Source: CAD feature listing. Evaluate the final solid. Frame: model axes, mm. A direction names the side the tool comes from. Give positions to 0.01 mm unless a question says otherwise; leave off trailing zeros. Write each loop counter-clockwise with the first axis right and the second up, starting at its lowest first coordinate (ties: lowest second). Pieces come first, ordered by that corner, then holes. Notation, with made-up numbers: M 10.25,85.5 L 58.25,85.5 A25 cw 58.25,107.5 Z; hole C 83,4 d4. An arc over 180 degrees is marked long. Answer as a JSON object with one key per item and string values. Group by question number.
```python
from build123d import *

# Parameters (mm, degrees)
SKETCH1_R           = 40
SKETCH1_R_2         = 25
BOSS_EXTRUDE1_DEPTH = 30
BOSS_EXTRUDE2_DEPTH = 17
SKETCH3_R           = 17.5
CUT_EXTRUDE1_DEPTH  = 181.856296545
CUT_EXTRUDE2_DEPTH  = 185.661853126
SKETCH6_R           = 4.5
CUT_EXTRUDE3_DEPTH  = 24


with BuildPart() as part:
    # Sketch1 → Boss-Extrude1 (new, symmetric)
    with BuildSketch(Plane(origin=(0, 0, 0), x_dir=(0, 0, -1), z_dir=(1, 0, 0))):
        Circle(SKETCH1_R)
        Circle(SKETCH1_R_2, mode=Mode.SUBTRACT)
    extrude(amount=BOSS_EXTRUDE1_DEPTH, both=True)

    # Sketch2 → Boss-Extrude2 (add, symmetric)
    with BuildSketch(Plane(origin=(0, 0, 0), x_dir=(0, 0, -1), z_dir=(1, 0, 0))):
        with BuildLine():
            Line((-19.364916731, 35), (-141.236028691, 29.974526403))
            ThreePointArc((-141.236028691, 29.974526403), (-170, 0), (-141.236028691, -29.974526403))
            Line((-141.236028691, -29.974526403), (-19.364916731, -35))
            ThreePointArc((-19.364916731, -35), (-40, 0), (-19.364916731, 35))
        make_face()
    extrude(amount=BOSS_EXTRUDE2_DEPTH, both=True)

    # Sketch3 → Cut-Extrude1 (cut, through all)
    with BuildSketch(Plane(origin=(17, 0, 0), x_dir=(0, 0, -1), z_dir=(1, 0, 0))):
        with Locations((-140, 0)):
            Circle(SKETCH3_R)
    extrude(amount=-CUT_EXTRUDE1_DEPTH, mode=Mode.SUBTRACT)

    # Sketch5 → Cut-Extrude2 (cut, through all)
    with BuildSketch(Plane(origin=(30, 0, 0), x_dir=(0, 0, -1), z_dir=(1, 0, 0))):
        Polygon((-3.702856162, 6.196638775), (-25.314422766, -15.41492783), (-15.41492783, -25.314422766), (6.196638775, -3.702856162), align=None)
    extrude(amount=-CUT_EXTRUDE2_DEPTH, mode=Mode.SUBTRACT)

    # Sketch6 → Cut-Extrude3 (cut)
    with BuildSketch(Plane.XY.offset(-35)):
        with Locations(Location((0, 0, 0), (0, 0, 180))):
            Circle(SKETCH6_R)
    extrude(amount=CUT_EXTRUDE3_DEPTH, mode=Mode.SUBTRACT)


solid = part.part
```
(1) Contact query for flat-ended pins moving along their axis: pin 1 Ø12 at (x, y) = (18, 8.5) entering from -Z; pin 2 Ø4 at (x, y) = (-14, 25.5) entering from +Z; pin 3 Ø4 at (x, y) = (-4.5, -20) entering from -Z. Output: stop coordinate, or through.
(2) Section C-C, the plane y = 12.5. Return loops of the section in (x, z).
(3) Section D-D, the plane x = -24. Return loops of the section in (y, z), plus the area to 3 significant figures.
(4) Pull-direction query (Z, two-part tool) for faces 1 (the flat face through (0, 0, -35)), 2 (the flat face through (-17, 0, 96)), 3 (the flat face through (0.238, 32.522, 79.447)); classes: pulls with the +Z half, pulls with the -Z half, needs draft (parallel to the pull), parting line crosses it, or undercut.
(5) Access query for faces 4 (the flat face through (-30, 18.34, -17.22)), 5 (the flat face through (0.42, -20.3, 20.43)), 6 (the cylindrical face through (3.6, 2.7, -29.9)). Directions: +Z, -Z, +X, -X, +Y, -Y. A direction counts if a zero-diameter tool reaches every point of the face in a straight line with its end or side. Return the directions, or none.
(6) Section A-A, the plane z = 0. Return loops of the section in (x, y), plus the area to 3 significant figures.
(7) Ray query, L1, parallel to Z at x = -8, y = 0.5 (3 decimals); L2, parallel to Y at x = -13, z = 0; L3, parallel to X at y = -22, z = 116. Return the intervals inside material, ascending. Write a range as [from, to].
(8) Section B-B, the plane x = 0. Return loops of the section in (y, z), plus the area to 3 significant figures.
Reported:
{
 "1": {"pin 1": "stops at z = -39.92", "pin 2": "stops at z = 158.65", "pin 3": "stops at z = -35.72"},
 "2": {"outline": "M -30,-38 L 30,-38 L 30,-21.65 L -30,-21.65 Z; M -30,21.65 L 30,21.65 L 30,38 L 17,38 L 17,127.75 L -17,127.75 L -17,38 L -30,38 Z; M -17,152.25 L 17,152.25 L 17,167.27 L -17,167.27 Z"},
 "3": {"outline": "C 0,0 d80; hole M -25.31,15.41 L -21.92,12.02 A25 ccw long -12.02,21.92 L -15.41,25.31 Z", "area": "3,010 mm2"},
 "4": {"face 1": "undercut", "face 2": "needs draft", "face 3": "pulls with the +Z half"},
 "5": {"face 4": "+Z, -Z, -X, +Y, -Y", "face 5": "+X, -X", "face 6": "none"},
 "6": {"outline": "M -30,-40 L 30,-40 L 30,-25 L -30,-25 Z; M -30,25 L 30,25 L 30,40 L -30,40 Z", "area": "1,800 mm2"},
 "7": {"L1": "z = [-39.997, -24.995], [24.995, 122.507], [157.493, 169.996]", "L2": "y = [-40, -25], [25, 40]", "L3": "x = [-17, 17]"},
 "8": {"outline": "M -35,19.36 A40 ccw long 35,19.36 L 29.97,141.24 A30 ccw -29.97,141.24 Z; hole M -25.31,15.41 L -21.92,12.02 A25 ccw -4.5,-24.59 L -4.5,-35 L 4.5,-35 L 4.5,-24.59 A25 ccw long -12.02,21.92 L -15.41,25.31 Z; hole C 0,140 d35", "area": "10,200 mm2"}
}
